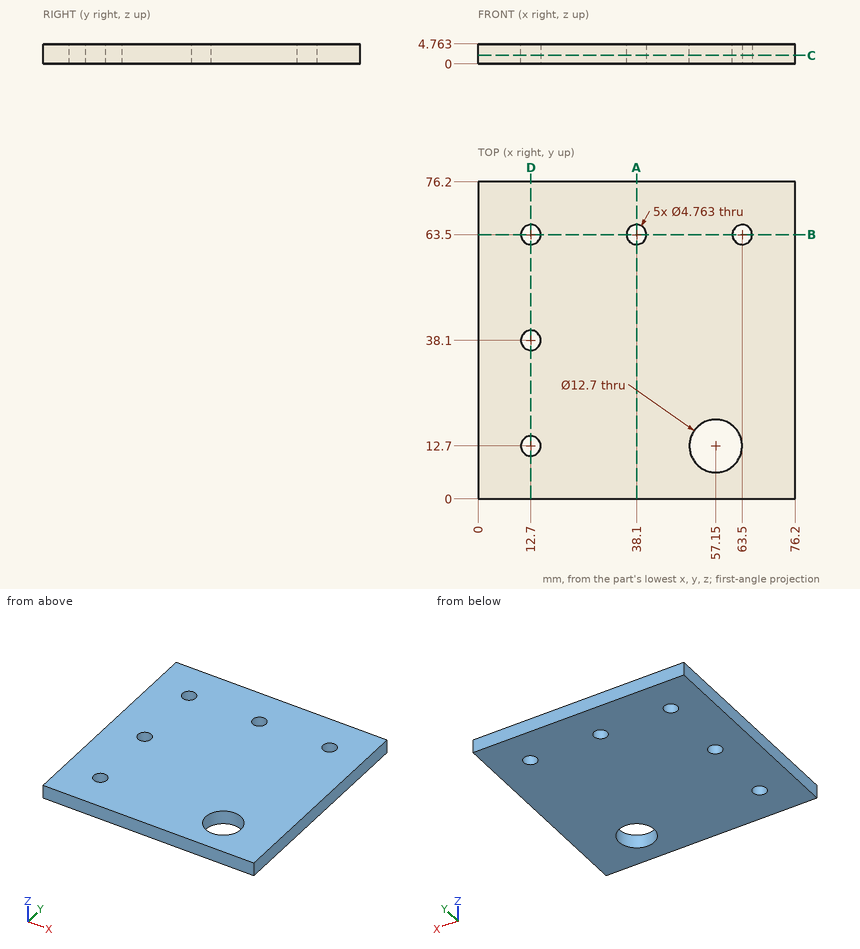
Drawing for the job (mm, zero at the part's lowest x, y, z). Round coordinates to 2 decimals unless told otherwise and drop trailing zeros. Write each loop counter-clockwise with the first axis right and the second up, starting at its lowest first coordinate (ties: lowest second). Pieces come first, ordered by that corner, then holes. Notation, with made-up numbers: M -14.5,21 L 20.5,21 A29 cw 20.5,46 Z; hole C -38.75,58.5 d11. An arc over 180 degrees is marked long. Answer in a Markdown table with one row per item.
1. Saw through at B-B (y = 63.5). List the corners of the cut face in (x, z).
Geometry check:
| item | result |
|---|---|
| outline | M 0,0 L 10.32,0 L 10.32,4.76 L 0,4.76 Z; M 15.08,0 L 35.72,0 L 35.72,4.76 L 15.08,4.76 Z; M 40.48,0 L 61.12,0 L 61.12,4.76 L 40.48,4.76 Z; M 65.88,0 L 76.2,0 L 76.2,4.76 L 65.88,4.76 Z |
2. Saw through at A-A (x = 38.1). List the corners of the cut face in (y, z).
Geometry check:
| item | result |
|---|---|
| outline | M 0,0 L 61.12,0 L 61.12,4.76 L 0,4.76 Z; M 65.88,0 L 76.2,0 L 76.2,4.76 L 65.88,4.76 Z |
3. Saw through at C-C (z = 2.05). List the corners of the cut face in (x, y), and give its area (3 significant figures).
Geometry check:
| item | result |
|---|---|
| outline | M 0,0 L 76.2,0 L 76.2,76.2 L 0,76.2 Z; hole C 12.7,12.7 d4.76; hole C 12.7,38.1 d4.76; hole C 12.7,63.5 d4.76; hole C 38.1,63.5 d4.76; hole C 57.15,12.7 d12.7; hole C 63.5,63.5 d4.76 |
| area | 5,590 mm2 |
4. Probe L1, parallel to Y at x = 12.7, z = 2.9; L2, parallel to Y at x = 12, z = 2.5 (1 decimal); L3, parallel to X at y = 63, z = 1. List the from-to ranges inside material, lowest first. Write a range as [from, to].
Geometry check:
| item | result |
|---|---|
| L1 | [0, 10.32], [15.08, 35.72], [40.48, 61.12], [65.88, 76.2] |
| L2 | [0, 10.4], [15, 35.8], [40.4, 61.2], [65.8, 76.2] |
| L3 | [0, 10.37], [15.03, 35.77], [40.43, 61.17], [65.83, 76.2] |
